The listing builds one solid part. Answer for the finished solid, in the listing's coordinates (mm). A direction names the side the tool comes from. Give positions to 0.01 mm unless a question says otherwise; leave off trailing zeros. Write each loop counter-clockwise with the first axis right and the second up, starting at its lowest first coordinate (ties: lowest second). Pieces come first, ordered by that corner, then holes. Notation, with made-up numbers: (9.25, 23) - (34.25, 23) arc R23 cw to (34.25, 54) - close; hole circle Ø10 at (30, 46.25). An arc over 180 degrees is marked (long way). Answer in a Markdown table with one row per item. Add a question column.
Autodesk Inventor part; units mm, degrees
ref_plane "YZ Plane" through (0, 0, 0) normal (1, 0, 0) x (0, 1, 0)
ref_plane "XZ Plane" through (0, 0, 0) normal (0, 1, 0) x (-1, 0, 0)
ref_plane "XY Plane" through (0, 0, 0) normal (0, 0, 1) x (1, 0, 0)
sketch "Sketch1" plane through (0, 0, 0) normal (0, 1, 0) x (-1, 0, 0)
  line L0 (0, 0) -> (-50.8, 0)
  line L1 (-50.8, 0) -> (-50.8, 44.45)
  line L2 (-50.8, 44.45) -> (0, 44.45)
  line L3 (0, 44.45) -> (0, 0)
  dimension "d0" = 44.45
  dimension "d1" = 50.8
extrude "Extrusion1" add sketch "Sketch1" along normal blind 3.175
sketch "Sketch2" plane through (0, 3.175, 0) normal (0, 1, 0) x (1, 0, 0)
  line L0 (50.8, 0) -> (0, 0)
  line L1 (0, 0) -> (0, -44.45)
  line L2 (0, -44.45) -> (50.8, -44.45)
  line L3 (50.8, -44.45) -> (50.8, 0)
  line L4 (3.175, -3.175) -> (47.625, -3.175)
  line L5 (47.625, -3.175) -> (47.625, -41.275)
  line L6 (47.625, -41.275) -> (3.175, -41.275)
  line L7 (3.175, -41.275) -> (3.175, -3.175)
  dimension "d4" = 3.175
  dimension "d5" = 3.175
  dimension "d6" = 3.175
  dimension "d7" = 3.175
extrude "Extrusion2" add sketch "Sketch2" along normal blind 6.35
sketch "Sketch3" plane through (0, 3.175, 0) normal (0, 1, 0) x (1, 0, 0)
  line L0 (47.625, -41.275) -> (47.625, -3.175)
  line L1 (47.625, -3.175) -> (3.175, -3.175)
  line L2 (3.175, -3.175) -> (3.175, -41.275)
  line L3 (3.175, -41.275) -> (47.625, -41.275)
  circle A0 centre (6.35, -38.1) radius 1.5875
  circle A1 centre (6.35, -6.35) radius 1.5875
  circle A2 centre (44.45, -6.35) radius 1.5875
  circle A3 centre (44.45, -38.1) radius 1.5875
  point P0 (0, 0)
  dimension "d10" = 3.175
  dimension "d11" = 3.175
  dimension "d12" = 3.175
  dimension "d13" = 3.175
  dimension "d14" = 3.175
  dimension "d15" = 3.175
  dimension "d16" = 3.175
  dimension "d17" = 3.175
  dimension "d18" = 3.175
  dimension "d19" = 3.175
  dimension "d20" = 3.175
  dimension "d21" = 3.175
extrude "Extrusion3" add sketch "Sketch3" along normal blind 12.7 contours A0 | A1 | A2 | A3
sketch "Sketch4" plane through (0, 0, 44.45) normal (0, 0, 1) x (1, 0, 0)
  line L0 (0, 9.525) -> (50.8, 9.525)
  line L1 (0, 0) -> (0, 9.525)
  line L2 (28.575, 9.525) -> (41.275, 9.525)
  line L3 (41.275, 9.525) -> (41.275, 3.175)
  line L4 (41.275, 3.175) -> (28.575, 3.175)
  line L5 (28.575, 3.175) -> (28.575, 9.525)
  dimension "d24" = 6.35
  dimension "d25" = 28.575
  dimension "d27" = 41.275
extrude "Extrusion4" cut sketch "Sketch4" against normal blind 3.175
sketch "Sketch5" plane through (50.8, 0, 44.45) normal (1, 0, 0) x (0, 0, -1)
  line L0 (0, 9.525) -> (44.45, 9.525)
  line L1 (0, 0) -> (0, 9.525)
  line L2 (12.7, 9.525) -> (25.4, 9.525)
  line L3 (25.4, 9.525) -> (25.4, 3.175)
  line L4 (25.4, 3.175) -> (12.7, 3.175)
  line L5 (12.7, 3.175) -> (12.7, 9.525)
  dimension "d30" = 12.7
  dimension "d31" = 25.4
  dimension "d32" = 6.35
extrude "Extrusion5" cut sketch "Sketch5" against normal blind 3.175
sketch "Sketch6" plane through (0, 3.175, 0) normal (0, 1, 0) x (1, 0, 0)
  circle A0 centre (44.45, -6.35) radius 1.5875
  circle A1 centre (6.35, -38.1) radius 1.5875
  circle A2 centre (6.35, -6.35) radius 1.5875
  circle A3 centre (44.45, -38.1) radius 1.5875
  line L0 (47.625, -41.275) -> (47.625, -31.75)
  line L1 (50.8, -31.75) -> (47.625, -31.75)
  line L2 (50.8, -19.05) -> (50.8, -31.75)
  line L3 (50.8, -19.05) -> (47.625, -19.05)
  line L4 (47.625, -19.05) -> (47.625, -3.175)
  line L5 (47.625, -3.175) -> (3.175, -3.175)
  line L6 (3.175, -3.175) -> (3.175, -41.275)
  line L7 (3.175, -41.275) -> (28.575, -41.275)
  line L8 (28.575, -44.45) -> (28.575, -41.275)
  line L9 (41.275, -44.45) -> (28.575, -44.45)
  line L10 (41.275, -44.45) -> (41.275, -41.275)
  line L11 (41.275, -41.275) -> (47.625, -41.275)
  point P0 (0, 0)
properties part number "Casing Bottom"
1. Straight lines are drawn through the part: L1, parallel to X at y = 6.5, z = 10 (3 decimals); L2, parallel to X at y = 12.25, z = 6.5; L3, parallel to Z at x = 10.5, y = 9 (3 decimals). For each, find the intervals that lie inside material, in ascending order. Write a range as [from, to].
2. The mould has two halves that part along X. Classify faces 1 (the face through (25, 6, 3.175)), 2 (the face through (26, 5, 44.45)), 3 (the face through (0, 5, 23)): +X half, -X half, draft (parallel to the pull), parting line (faces both ways), or undercut.
3. A tool of negligible diameter and unlimited length cuts with its end or side. For faces 4 (the face through (28.575, 6, 43)), 5 (the face through (6, 15.875, 38)), 6 (the face through (49, 6, 19.05)), 7 (the face through (48, 9.525, 39)), 8 (the face through (47.625, 6, 11)), from which of +Z, -Z, +X, -X, +Y, -Y can it reach the whole face along a straight path? Write none if from no direction.
4. Section C-C (z = 29.5) is taken. Give the vertices of the cut face in (x, y) (3 decimals).
5. Given pin 1 Ø2 at (x, y) = (10, 13.5) entering from +Z; pin 2 Ø7 at (y, z) = (6.5, 12.5) entering from -X; pin 3 Ø13.5 at (x, z) = (30.5, 25) entering from +Y (3 decimals); pin 4 Ø4 at (y, z) = (12.5, 39.5) entering from +X, each flat-ended and moving along its own axis, determine where each tip first touches the part or whether it passes through.
6. Section B-B (x = 35.5) is taken. Give the vertices of the cut face in (y, z) (3 decimals).
7. Section A-A (y = 7.5) is taken. State how many separate pieces and enclosed holes the cut face has, and give its area (3 significant figures).
Geometry check:
| question | item | result |
|---|---|---|
| 1 | L1 | [0, 3.175], [47.625, 50.8] |
| 1 | L2 | [4.77, 7.93], [42.87, 46.03] |
| 1 | L3 | [0, 3.175], [41.275, 44.45] |
| 2 | face 1 | undercut |
| 2 | face 2 | draft |
| 2 | face 3 | -X half |
| 3 | face 4 | +Z, +Y |
| 3 | face 5 | +Z, -Z, +X, -X, +Y |
| 3 | face 6 | +X, +Y |
| 3 | face 7 | +Z, +X, +Y |
| 3 | face 8 | +Y |
| 4 | outline | (0, 0) - (50.8, 0) - (50.8, 3.175) - (3.175, 3.175) - (3.175, 9.525) - (0, 9.525) - close |
| 5 | pin 1 | through |
| 5 | pin 2 | x = 0 |
| 5 | pin 3 | y = 3.175 |
| 5 | pin 4 | x = 46.04 |
| 6 | outline | (0, 0) - (9.525, 0) - (9.525, 3.175) - (3.175, 3.175) - (3.175, 44.45) - (0, 44.45) - close |
| 7 | separate pieces | 6 |
| 7 | enclosed holes | 0 |
| 7 | area | 516 mm² |
